from build123d import *

# Parameters (mm, degrees)
F1_DEPTH = 6.35
F2_R     = 3.175
F3_DEPTH = 25.4
F2_R_2   = 5.715
F4_DEPTH = 4.572


with BuildPart() as f1:
    # F0 (on Front) → F1 (new body)
    with BuildSketch(Plane.XZ):
        with BuildLine():
            ThreePointArc((-11.6955887006, 80.7483033067), (-2.5254725798, 63.3518676414), (12.7, 75.7982321005))
            ThreePointArc((12.7, 75.7982321005), (12.4463644591, 78.3237046803), (11.6955887006, 80.7483033067))
            ThreePointArc((11.6955887006, 80.7483033067), (0, 88.4982321005), (-11.6955887006, 80.7483033067))
        make_face()
        with BuildLine():
            ThreePointArc((11.6955887006, 80.7483033067), (12.4463644591, 78.3237046803), (12.7, 75.7982321005))
            ThreePointArc((12.7, 75.7982321005), (-2.5254725798, 63.3518676414), (-11.6955887006, 80.7483033067))
            Line((-11.6955887006, 80.7483033067), (-56.9148214828, 7.5573103616))
            ThreePointArc((-56.9148214828, 7.5573103616), (-42.7291164055, 12.06058246), (-34.0081050618, 0))
            ThreePointArc((-34.0081050618, 0), (-37.7278489407, -8.9802561211), (-46.7081050618, -12.7))
            Line((-46.7081050618, -12.7), (47.4196799213, -12.7))
            ThreePointArc((47.4196799213, -12.7), (36.3047725839, 6.1440080469), (58.1740232476, 6.7553015936))
            Line((58.1740232476, 6.7553015936), (11.6955887006, 80.7483033067))
        make_face()
        with BuildLine():
            Line((47.4196799213, -12.7), (58.1740232476, 6.7553015936))
            ThreePointArc((58.1740232476, 6.7553015936), (36.3047725839, 6.1440080469), (47.4196799213, -12.7))
        make_face()
        with BuildLine():
            ThreePointArc((60.1196799213, 0), (59.6235760255, 3.5149565969), (58.1740232476, 6.7553015936))
            Line((58.1740232476, 6.7553015936), (47.4196799213, -12.7))
            ThreePointArc((47.4196799213, -12.7), (56.3999360424, -8.9802561211), (60.1196799213, 0))
        make_face()
        with BuildLine():
            Line((-46.7081050618, -12.7), (-56.9148214828, 7.5573103616))
            ThreePointArc((-56.9148214828, 7.5573103616), (-58.0497945654, -5.7145497814), (-46.7081050618, -12.7))
        make_face()
        with BuildLine():
            ThreePointArc((-34.0081050618, 0), (-42.7291164055, 12.06058246), (-56.9148214828, 7.5573103616))
            Line((-56.9148214828, 7.5573103616), (-46.7081050618, -12.7))
            ThreePointArc((-46.7081050618, -12.7), (-37.7278489407, -8.9802561211), (-34.0081050618, 0))
        make_face()
    extrude(amount=F1_DEPTH)

    # F2 (on face) → F3 (cut)
    with BuildSketch(Plane.XZ.offset(6.35)):
        with Locations((-46.7081050618, 0)):
            Circle(F2_R)
        with Locations((47.4196799213, 0)):
            Circle(F2_R)
        with Locations((0, 75.7982321005)):
            Circle(F2_R)
    extrude(amount=-F3_DEPTH, mode=Mode.SUBTRACT)

    # F2 (on face) → F4 (join)
    with BuildSketch(Plane.XZ.offset(6.35)):
        with Locations((47.4196799213, 0)):
            Circle(F2_R_2)
        with Locations((47.4196799213, 0)):
            Circle(F2_R, mode=Mode.SUBTRACT)
        with Locations((-46.7081050618, 0)):
            Circle(F2_R_2)
        with Locations((-46.7081050618, 0)):
            Circle(F2_R, mode=Mode.SUBTRACT)
        with Locations((0, 75.7982321005)):
            Circle(F2_R_2)
        with Locations((0, 75.7982321005)):
            Circle(F2_R, mode=Mode.SUBTRACT)
    extrude(amount=F4_DEPTH)


solid = f1.part
For this review, take the finished solid that the model builds, in its own axes (mm). A direction names the side the tool comes from. Round coordinates to 2 decimals unless told otherwise and drop trailing zeros. Order: outer loops, then holes, each group sorted by start corner. A loop starts at its lowest first (then second) coordinate and runs counter-clockwise, first axis right, second up. Notation, with made-up numbers: M 51,26 L 80,26 A33 ccw 80,56 Z; hole C -18,-2.75 d6. An arc over 180 degrees is marked long. Use a Markdown table: item, result. Add a question column.
Item 1: Add section C-C, the plane x = 14. Give the boundary of the cut face in (y, z), then the cut area to 3 significant figures.
Item 2: Add section D-D, the plane z = 20. Give the boundary of the cut face in (x, y), then the cut area to 3 significant figures.
Item 3: Add section A-A, the plane x = 0. Give the boundary of the cut face in (y, z), then the cut area to 3 significant figures.
Item 4: Mouldability with a two-part tool opening along X and no side actions: class faces 1 (the cylindrical face through (-50.92, -8.6, 3.86)), 2 (the flat face through (0, -3, -12.7)), 3 (the cylindrical face through (41.71, -8.6, 0.25)), 4 (the cylindrical face through (-58.137, -3.131, -5.539)) as released by +X, released by -X, zero draft, split by the parting line, or undercut.
Item 5: Add section B-B, the plane y = -3.5. Give the boundary of the cut face in (x, z) (3 decimals), then the cut area to 3 significant figures.
Item 6: Insertion check: pin 1 (10 mm diameter, centred on x = 1, z = 34.5, fed in from -Y); pin 2 (1 mm diameter, centred on x = 5, z = 18.5, fed in from +Y); pin 3 (6 mm diameter, centred on y = -3.5, z = 60.5, fed in from -X). Each pin has a flat end and moves straight along its axis. Give the tip position at first contact, or say it passes through.
Item 7: Tool access review of faces 5 (the cylindrical face through (-0.744, -8.604, 81.465)), 6 (the flat face through (-44, -10.922, -2)): name each direction out of +Z, -Z, +X, -X, +Y, -Y from which nothing blocks a thin tool from reaching the whole face with its end or side.
Item 8: To check wall thickness, follow line 1 along X through (y, z) = (-1.25, -0.5); line 2 along Y through (x, z) = (-7.5, 64); line 3 along X through (y, z) = (-9.5, 76.5). State the ranges of each line that lie inside material, in increasing order.
Geometry results:
| question | item | result |
|---|---|---|
| 1 | outline | M -6.35,-12.7 L 0,-12.7 L 0,77.08 L -6.35,77.08 Z |
| 1 | area | 570 mm² |
| 2 | outline | M -49.23,-6.35 L 49.85,-6.35 L 49.85,0 L -49.23,0 Z |
| 2 | area | 629 mm² |
| 3 | outline | M -10.92,70.08 L -6.35,70.08 L -6.35,-12.7 L 0,-12.7 L 0,72.62 L -10.92,72.62 Z; M -10.92,78.97 L 0,78.97 L 0,88.5 L -6.35,88.5 L -6.35,81.51 L -10.92,81.51 Z |
| 3 | area | 626 mm² |
| 4 | face 1 | undercut |
| 4 | face 2 | zero draft |
| 4 | face 3 | undercut |
| 4 | face 4 | released by -X |
| 5 | outline | M -56.915,7.557 A12.7 ccw -46.708,-12.7 L 47.42,-12.7 A12.7 ccw 58.174,6.755 L 11.696,80.748 A12.7 ccw -11.696,80.748 Z; hole C -46.708,0 d6.35; hole C 0,75.798 d6.35; hole C 47.42,0 d6.35 |
| 5 | area | 7,430 mm² |
| 6 | pin 1 | stops at y = -6.35 |
| 6 | pin 2 | stops at y = 0 |
| 6 | pin 3 | stops at x = -26.06 |
| 7 | face 5 | -Y |
| 7 | face 6 | +Z, -Z, +X, -X, -Y |
| 8 | line 1 | x = -59.4 to -49.84, -43.57 to 44.28, 50.56 to 60.11 |
| 8 | line 2 | y = -6.35 to 0 |
| 8 | line 3 | x = -5.67 to -3.1, 3.1 to 5.67 |
